Design review of the part shown in the three views and the two pictorial views. Dimensions are in mm from the part's minimum x, y and z. A direction names the side the tool comes from. Round coordinates to 2 decimals unless told otherwise and drop trailing zeros. Write each loop counter-clockwise with the first axis right and the second up, starting at its lowest first coordinate (ties: lowest second). Pieces come first, ordered by that corner, then holes. Notation, with made-up numbers: (27, -9) - (74, -9) arc R30 cw to (74, 26) - close; hole circle Ø3 at (-40, 14.25). An arc over 180 degrees is marked (long way). Use one line per item in the form item = value.
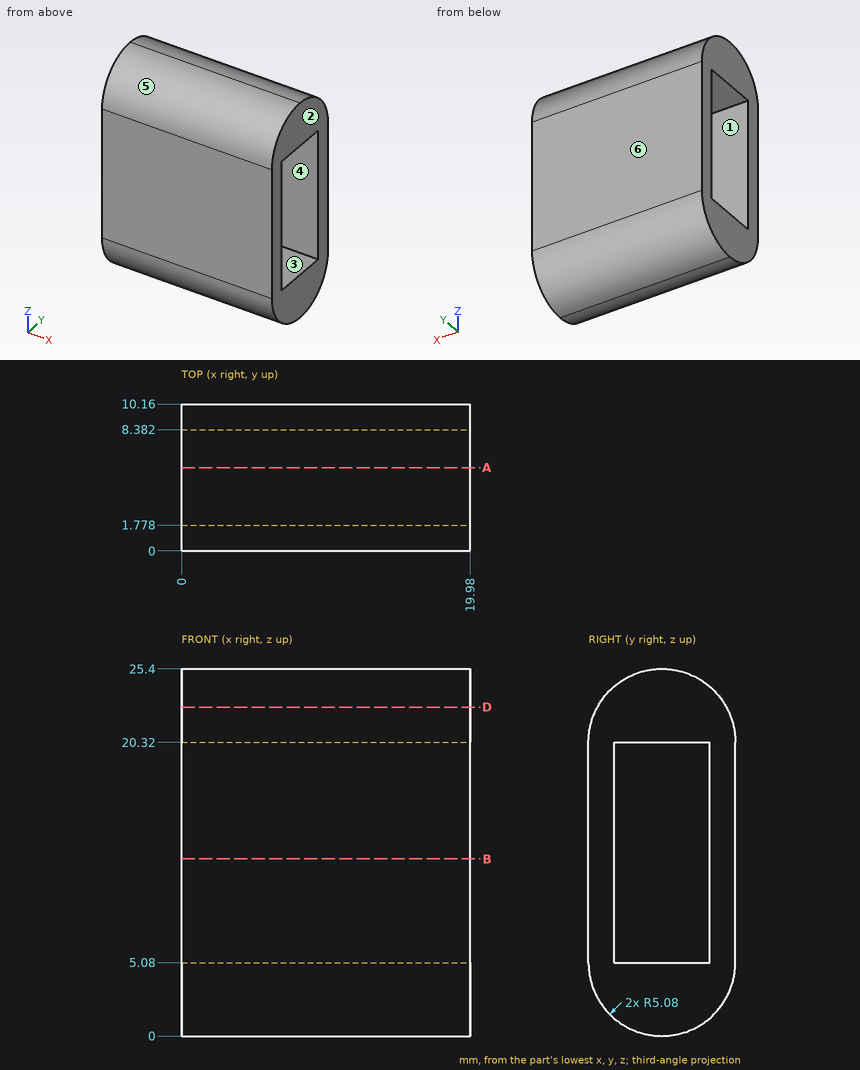
Q1. Draft analysis for pull direction Y (two halves, no side actions). For the marked faces 3, 4, 5 and 6, state which applies: released by +Y, released by -Y, zero draft, split by the parting line, or undercut.
Calculated:
face_3 = undercut
face_4 = undercut
face_5 = released by -Y
face_6 = released by +Y
Q2. We need section B-B on z = 12.25. Write out the cut boundary in (x, y).
Calculated:
outline = (0, 0) - (19.98, 0) - (19.98, 1.78) - (0, 1.78) - close; (0, 8.38) - (19.98, 8.38) - (19.98, 10.16) - (0, 10.16) - close
Q3. To check wall thickness, follow line 1 along Y through (x, z) = (11.25, 12.25); line 2 along Z through (x, y) = (4, 4); line 3 along Z through (x, y) = (18.5, 4.5). State the ranges of each line that lie inside material, in increasing order. Write a range as from..to.
Calculated:
line_1 = 0..1.78, 8.38..10.16
line_2 = 0.12..5.08, 20.32..25.28
line_3 = 0.03..5.08, 20.32..25.37
Q4. We need section A-A on y = 5.75. Write out the cut boundary in (x, z) (1 decimal), then the cut area to 3 significant figures.
Calculated:
outline = (0, 0) - (20, 0) - (20, 5.1) - (0, 5.1) - close; (0, 20.3) - (20, 20.3) - (20, 25.4) - (0, 25.4) - close
area = 201 mm2
Q5. Machinability: for the marked faces 1 and 2, which of the approach directions +Z, -Z, +X, -X, +Y, -Y give a long, thin tool a straight path to every point of the face, cutting with its end or side? Answer none if there is none.
Calculated:
face_1 = +X, -X
face_2 = +Z, -Z, +X, +Y, -Y
Q6. We need section D-D on z = 22.75. Write out the cut boundary in (x, y), then the cut area to 3 significant figures.
Calculated:
outline = (0, 0.62) - (19.98, 0.62) - (19.98, 9.54) - (0, 9.54) - close
area = 178 mm2
